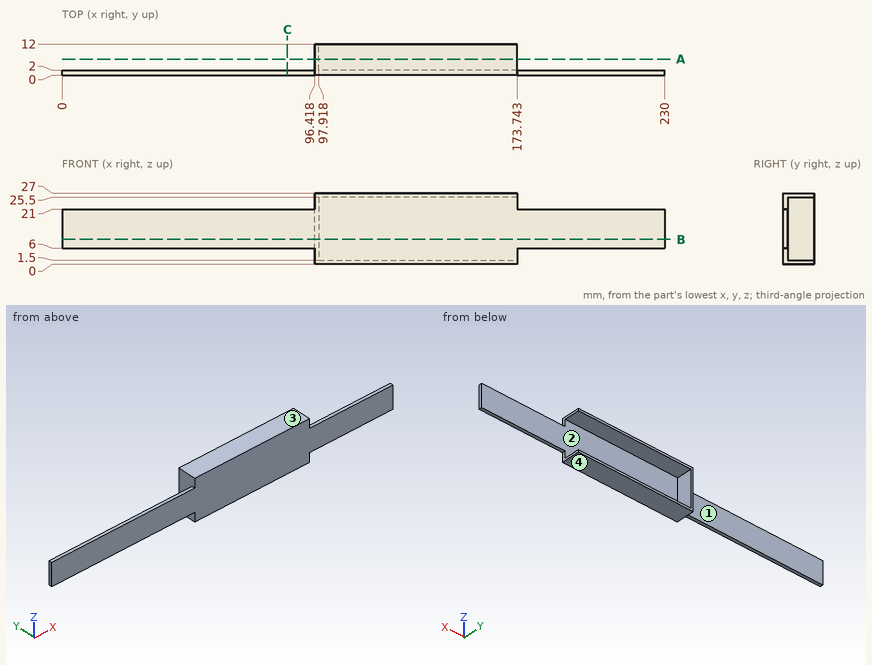
Print and shaded views of the part. All mm, measured from the part's lowest x, y and z. Coordinates: 2 decimals unless noted, no trailing zeros. Order: outer loops, then holes, each group sorted by start corner. A loop starts at its lowest first (then second) coordinate and runs counter-clockwise, first axis right, second up. Notation, with made-up numbers: M 66,53 L 89,53 A23 cw 89,61 Z; hole C 89,-22 d3. An arc over 180 degrees is marked long. Write each question's results on one line, items separated by ' | '. Start each with the question number.
Q1. Pull direction Z, two halves, no side cores. Call the marked faces 1, 2, 3 and 4: +Z half, -Z half, draft (parallel to the pull), parting line (faces both ways), or undercut.
Q2. Cut at B-B (z = 9.5). List the corners of the cut face in (x, y), then the cut area to 3 significant figures.
Q3. Drill centre lines: probe 1 along Z at (x, y) = (159.5, 7.5); probe 2 along X at (y, z) = (3, 1.75); probe 3 along Y at (x, z) = (103.5, 7.25). Where is each one in solid material? Low to high. Write a range as from..to.
Q4. Cut at C-C (x = 86). List the corners of the cut face in (y, z).
Q5. Cut at A-A (y = 6.25). List the corners of the cut face in (x, z).
Q6. Flat gauge pins, fed straight in: P1, Ø1, axis at x = 45, y = 0.5, coming from the -Z side; P2, Ø2, axis at x = 188, y = 1, coming from the +Z side; P3, Ø3, axis at y = 4, z = 2, coming from the +X side. Where does each tip first touch, or does it go through?
Found:
1) face 1: draft | face 2: undercut | face 3: +Z half | face 4: -Z half
2) outline: M 0,0 L 230,0 L 230,2 L 97.92,2 L 97.92,12 L 96.42,12 L 96.42,2 L 0,2 Z | area: 475 mm²
3) probe 1: 0..1.5, 25.5..27 | probe 2: 96.42..97.92 | probe 3: 0..2
4) outline: M 0,6 L 2,6 L 2,21 L 0,21 Z
5) outline: M 96.42,0 L 173.74,0 L 173.74,1.5 L 97.92,1.5 L 97.92,25.5 L 173.74,25.5 L 173.74,27 L 96.42,27 Z
6) P1: z = 6 | P2: z = 21 | P3: x = 173.74
